```python
from build123d import *

# Parameters (mm, degrees)
F1_DEPTH = 26
F2_SIZE2 = 16.336822
F2_SIZE  = 11.55


with BuildPart() as f1:
    # F0 (on Top) → F1 (new body)
    with BuildSketch(Plane.XY):
        Polygon((0, 92.376043), (-80, -46.188022), (80, -46.188022), align=None)
    extrude(amount=F1_DEPTH)

    # F2
    f2_edges = [f1.edges().sort_by_distance(p)[0] for p in [
        (-40, 23.094011, 26),
        (40, 23.094011, 26),
        (0, -46.188022, 26),
    ]]
    chamfer(f2_edges, length=F2_SIZE, length2=F2_SIZE2)


solid = f1.part
```
Verification items for the finished model (mm, model axes). Round coordinates to 2 decimals unless told otherwise and drop trailing zeros. Write each loop counter-clockwise with the first axis right and the second up, starting at its lowest first coordinate (ties: lowest second). Pieces come first, ordered by that corner, then holes. Notation, with made-up numbers: (12.25, -35) - (17.25, -35) arc R10 ccw to (17.25, -21) - close; hole circle Ø5 at (41.25, 63). An arc over 180 degrees is marked (long way). Answer as a JSON object with one key per item and string values. Group by question number.
Q1. Section check D-D, the plane y = 78. Enter the section's corners in (x, z), plus the area to 3 significant figures.
Q2. Section check A-A, the plane y = -21. Enter the section's corners in (x, z), plus the area to 3 significant figures.
Q3. Section check B-B, the plane x = 70. Enter the section's corners in (y, z).
Q4. Go/stop test with flat-tipped pins: pin 1 Ø12 at (y, z) = (66.5, 3) entering from -X; pin 2 Ø2 at (y, z) = (-11, 15) entering from +X; pin 3 Ø8 at (y, z) = (-30.5, 4) entering from -X. Record where each tip stops, or that it passes through.
Q5. Section check C-C, the plane z = 4.5. Enter the section's corners in (x, y), plus the area to 3 significant figures.
Q6. Thickness scan on line 1 (X direction, y = -11, z = 13.25); line 2 (Y direction, x = -9, z = 11.25); line 3 (Y direction, x = 20, z = 3). Record the ranges inside material, lowest first.
Found:
{
 "1": {"outline": "(-8.3, 0) - (8.3, 0) - (8.3, 14.45) - (0, 19.53) - (-8.3, 14.45) - close", "area": "282 mm^2"},
 "2": {"outline": "(-65.46, 0) - (65.46, 0) - (65.46, 14.45) - (46.59, 26) - (-46.59, 26) - (-65.46, 14.45) - close", "area": "3,190 mm^2"},
 "3": {"outline": "(-46.19, 0) - (-28.87, 0) - (-28.87, 14.45) - (-40.41, 18.53) - (-46.19, 14.45) - close"},
 "4": {"pin 1": "stops at x = -18.4", "pin 2": "stops at x = 60.17", "pin 3": "stops at x = -73.25"},
 "5": {"outline": "(-80, -46.19) - (80, -46.19) - (0, 92.38) - close", "area": "11,100 mm^2"},
 "6": {"line 1": "x = -59.68 to 59.68", "line 2": "y = -46.19 to 76.79", "line 3": "y = -46.19 to 57.74"}
}
